```python
from build123d import *

# Parameters (mm, degrees)
BOSS_EXTRUDE2_DEPTH = 4
CUT_EXTRUDE2_REACH  = 8.5
SKETCH3_R           = 0.205
SHELL1_T            = -0.25


with BuildPart() as part:
    # Sketch1 → Boss-Extrude2 (new body, symmetric)
    with BuildSketch(Plane.XY):
        with BuildLine():
            Line((-7.485975276, 0), (-4.875, 0))
            ThreePointArc((-4.875, 0), (0, -4.875), (4.875, 0))
            Line((4.875, 0), (7.485975276, 0))
            Line((7.485975276, 0), (7.485975276, -0.41))
            Line((7.485975276, -0.41), (5.985975276, -0.41))
            ThreePointArc((5.985975276, -0.41), (5.186676874, -3.016352599), (3.31662479, -5))
            Line((3.31662479, -5), (7, -5))
            Line((7, -5), (7, -6.5))
            Line((7, -6.5), (-7, -6.5))
            Line((-7, -6.5), (-7, -5))
            Line((-7, -5), (-3.31662479, -5))
            ThreePointArc((-3.31662479, -5), (-5.186676874, -3.016352599), (-5.985975276, -0.41))
            Line((-5.985975276, -0.41), (-7.485975276, -0.41))
            Line((-7.485975276, -0.41), (-7.485975276, 0))
        make_face()
    extrude(amount=BOSS_EXTRUDE2_DEPTH, both=True)

    # Sketch3 → Cut-Extrude2 (cut, up to next)
    with BuildSketch(Plane(origin=(0, 0, 0), x_dir=(1, 0, 0), z_dir=(0, 1, 0)), mode=Mode.PRIVATE) as cut_extrude2_sk1:
        with Locations((-6.735975276, 3)):
            Circle(SKETCH3_R)
    cut_extrude2_tool1 = extrude(cut_extrude2_sk1.sketch, amount=-CUT_EXTRUDE2_REACH, mode=Mode.PRIVATE) & part.part
    add(cut_extrude2_tool1.solids().sort_by_distance((-6.735975, 0, -3))[0], mode=Mode.SUBTRACT)
    # Sketch3 → Cut-Extrude2 (cut, up to next)
    with BuildSketch(Plane(origin=(0, 0, 0), x_dir=(1, 0, 0), z_dir=(0, 1, 0)), mode=Mode.PRIVATE) as cut_extrude2_sk2:
        with Locations((-6.735975276, 1)):
            Circle(SKETCH3_R)
    cut_extrude2_tool2 = extrude(cut_extrude2_sk2.sketch, amount=-CUT_EXTRUDE2_REACH, mode=Mode.PRIVATE) & part.part
    add(cut_extrude2_tool2.solids().sort_by_distance((-6.735975, 0, -1))[0], mode=Mode.SUBTRACT)
    # Sketch3 → Cut-Extrude2 (cut, up to next)
    with BuildSketch(Plane(origin=(0, 0, 0), x_dir=(1, 0, 0), z_dir=(0, 1, 0)), mode=Mode.PRIVATE) as cut_extrude2_sk3:
        with Locations((-6.735975276, -1)):
            Circle(SKETCH3_R)
    cut_extrude2_tool3 = extrude(cut_extrude2_sk3.sketch, amount=-CUT_EXTRUDE2_REACH, mode=Mode.PRIVATE) & part.part
    add(cut_extrude2_tool3.solids().sort_by_distance((-6.735975, 0, 1))[0], mode=Mode.SUBTRACT)
    # Sketch3 → Cut-Extrude2 (cut, up to next)
    with BuildSketch(Plane(origin=(0, 0, 0), x_dir=(1, 0, 0), z_dir=(0, 1, 0)), mode=Mode.PRIVATE) as cut_extrude2_sk4:
        with Locations((-6.735975276, -3)):
            Circle(SKETCH3_R)
    cut_extrude2_tool4 = extrude(cut_extrude2_sk4.sketch, amount=-CUT_EXTRUDE2_REACH, mode=Mode.PRIVATE) & part.part
    add(cut_extrude2_tool4.solids().sort_by_distance((-6.735975, 0, 3))[0], mode=Mode.SUBTRACT)
    # Sketch3 → Cut-Extrude2 (cut, up to next)
    with BuildSketch(Plane(origin=(0, 0, 0), x_dir=(1, 0, 0), z_dir=(0, 1, 0)), mode=Mode.PRIVATE) as cut_extrude2_sk5:
        with Locations((6.735975276, -3)):
            Circle(SKETCH3_R)
    cut_extrude2_tool5 = extrude(cut_extrude2_sk5.sketch, amount=-CUT_EXTRUDE2_REACH, mode=Mode.PRIVATE) & part.part
    add(cut_extrude2_tool5.solids().sort_by_distance((6.735975, 0, 3))[0], mode=Mode.SUBTRACT)
    # Sketch3 → Cut-Extrude2 (cut, up to next)
    with BuildSketch(Plane(origin=(0, 0, 0), x_dir=(1, 0, 0), z_dir=(0, 1, 0)), mode=Mode.PRIVATE) as cut_extrude2_sk6:
        with Locations((6.735975276, -1)):
            Circle(SKETCH3_R)
    cut_extrude2_tool6 = extrude(cut_extrude2_sk6.sketch, amount=-CUT_EXTRUDE2_REACH, mode=Mode.PRIVATE) & part.part
    add(cut_extrude2_tool6.solids().sort_by_distance((6.735975, 0, 1))[0], mode=Mode.SUBTRACT)
    # Sketch3 → Cut-Extrude2 (cut, up to next)
    with BuildSketch(Plane(origin=(0, 0, 0), x_dir=(1, 0, 0), z_dir=(0, 1, 0)), mode=Mode.PRIVATE) as cut_extrude2_sk7:
        with Locations((6.735975276, 1)):
            Circle(SKETCH3_R)
    cut_extrude2_tool7 = extrude(cut_extrude2_sk7.sketch, amount=-CUT_EXTRUDE2_REACH, mode=Mode.PRIVATE) & part.part
    add(cut_extrude2_tool7.solids().sort_by_distance((6.735975, 0, -1))[0], mode=Mode.SUBTRACT)
    # Sketch3 → Cut-Extrude2 (cut, up to next)
    with BuildSketch(Plane(origin=(0, 0, 0), x_dir=(1, 0, 0), z_dir=(0, 1, 0)), mode=Mode.PRIVATE) as cut_extrude2_sk8:
        with Locations((6.735975276, 3)):
            Circle(SKETCH3_R)
    cut_extrude2_tool8 = extrude(cut_extrude2_sk8.sketch, amount=-CUT_EXTRUDE2_REACH, mode=Mode.PRIVATE) & part.part
    add(cut_extrude2_tool8.solids().sort_by_distance((6.735975, 0, -3))[0], mode=Mode.SUBTRACT)

    # Shell1
    shell1_openings = [part.faces().sort_by_distance(p)[0] for p in [
        (-6.735975276, 0, -0.795),
        (0, -2.4375, 0),
        (6.735975276, 0, 2.795),
    ]]
    offset(amount=SHELL1_T, openings=shell1_openings, kind=Kind.INTERSECTION)


solid = part.part
```
Input: part model. Units: mm. Frame: model coordinates. A direction names the side the tool comes from. Give positions to 0.01 mm unless a question says otherwise; leave off trailing zeros. Order: outer loops, then holes, each group sorted by start corner. A loop starts at its lowest first (then second) coordinate and runs counter-clockwise, first axis right, second up. Notation, with made-up numbers: (72, 50.5) - (102, 50.5) arc R14 cw to (102, 54.5) - close; hole circle Ø4 at (59, 23.25). An arc over 180 degrees is marked (long way). Use a Markdown table: item, result.
(1) Section query D-D (z = -3). State how many separate pieces and enclosed holes the cut face has, then the cut area to 3 significant figures.
Computed values:
| item | result |
|---|---|
| separate pieces | 3 |
| enclosed holes | 0 |
| area | 9.89 mm2 |
(2) Line query: line 1 (X direction, y = -0.25, z = -3); line 2 (Z direction, x = -5.25, y = -0.5); line 3 (Y direction, x = -6.5, z = -2.5). Output: solid intervals per line, ascending. Write a range as from..to.
Computed values:
| item | result |
|---|---|
| line 1 | x = -7.49..-6.94, -6.53..-5.74, 5.74..6.53, 6.94..7.49 |
| line 2 | z = -4..-3.75, 3.75..4 |
| line 3 | y = -6.5..-6.25, -5.25..-5, -0.41..-0.16 |
(3) Draft query along Z for faces 1 (the flat face through (5, -5, 0)), 2 (the flat face through (0.1, -5.4, 4)), 3 (the flat face through (-5, -5.25, 0)). Return one class per face: released by +Z, released by -Z, zero draft, split by the parting line, or undercut.
Computed values:
| item | result |
|---|---|
| face 1 | zero draft |
| face 2 | released by +Z |
| face 3 | undercut |
(4) Pin query (flat end, axial travel): pin 1 (4 mm diameter, centred on x = -5.5, z = -0.5, fed in from +Y); pin 2 (1.5 mm diameter, centred on y = -4.5, z = 1.5, fed in from +X); pin 3 (4 mm diameter, centred on x = 1.5, z = -1, fed in from +Y); pin 4 (1.1 mm diameter, centred on x = 5.5, z = -0.5, fed in from +Y). Return the tip coordinate at first contact, or that it passes through.
Computed values:
| item | result |
|---|---|
| pin 1 | stops at y = 0 |
| pin 2 | stops at x = 7 |
| pin 3 | stops at y = -4.56 |
| pin 4 | stops at y = -0.16 |
(5) Section query C-C (x = 0). Output: boundary loops of the cut face in (y, z) (3 decimals).
Computed values:
| item | result |
|---|---|
| outline | (-6.5, -4) - (-4.875, -4) - (-4.875, -3.75) - (-6.25, -3.75) - (-6.25, 3.75) - (-4.875, 3.75) - (-4.875, 4) - (-6.5, 4) - close |
(6) Access query for faces 4 (the cylindrical face through (4.805, -3.158, 0.053)), 5 (the flat face through (7, -6, 0)), 6 (the flat face through (0, -6.25, 0)). Directions: +Z, -Z, +X, -X, +Y, -Y. A direction counts if a zero-diameter tool reaches every point of the face in a straight line with its end or side. Return the directions, or none.
Computed values:
| item | result |
|---|---|
| face 4 | +Y |
| face 5 | +Z, -Z, +X, -Y |
| face 6 | none |
(7) Section query A-A (y = -1.5). Output: boundary loops of the cut face in (x, z), then the cut area to 3 significant figures.
Computed values:
| item | result |
|---|---|
| outline | (-5.81, -4) - (-4.64, -4) - (-4.64, -3.75) - (-5.55, -3.75) - (-5.55, 3.75) - (-4.64, 3.75) - (-4.64, 4) - (-5.81, 4) - close; (4.64, -4) - (5.81, -4) - (5.81, 4) - (4.64, 4) - (4.64, 3.75) - (5.55, 3.75) - (5.55, -3.75) - (4.64, -3.75) - close |
| area | 5.05 mm2 |
(8) Section query B-B (z = -1.75). Output: boundary loops of the cut face in (x, y), then the cut area to 3 significant figures.
Computed values:
| item | result |
|---|---|
| outline | (-7.49, -0.41) - (-5.99, -0.41) arc R6 ccw to (-3.32, -5) - (-7, -5) - (-7, -6.5) - (7, -6.5) - (7, -5) - (3.32, -5) arc R6 ccw to (5.99, -0.41) - (7.49, -0.41) - (7.49, 0) - (7.24, 0) - (7.24, -0.16) - (5.75, -0.16) arc R5.75 cw to (2.35, -5.25) - (6.75, -5.25) - (6.75, -6.25) - (-6.75, -6.25) - (-6.75, -5.25) - (-2.35, -5.25) arc R5.75 cw to (-5.75, -0.16) - (-7.24, -0.16) - (-7.24, 0) - (-7.49, 0) - close |
| area | 9.94 mm2 |
